from build123d import *

# Parameters (mm, degrees)
F0_W     = 711.2
F0_H     = 254
F1_DEPTH = 457.2
F3_DEPTH = 711.201
F4_R     = 19.05


with BuildPart() as f1:
    # F0 (on Top) → F1 (new body)
    with BuildSketch(Plane.XY):
        Rectangle(F0_W, F0_H)
    extrude(amount=F1_DEPTH)

    # F2 (on face) → F3 (cut, through all)
    with BuildSketch(Plane.YZ.offset(355.6)):
        Polygon((-127, 457.2), (-127, 0), (0, 457.2), align=None)
    extrude(amount=-F3_DEPTH, mode=Mode.SUBTRACT)

    # F4
    f4_edges = [f1.edges().sort_by_distance(p)[0] for p in [
        (0, -127, 0),
        (355.6, 0, 0),
        (355.6, -63.5, 228.6),
        (-355.6, -63.5, 228.6),
        (-355.6, 0, 0),
        (-355.6, 63.5, 457.2),
        (0, 0, 457.2),
        (355.6, 63.5, 457.2),
        (355.6, 127, 228.6),
        (0, 127, 0),
        (-355.6, 127, 228.6),
        (0, 127, 457.2),
    ]]
    fillet(f4_edges, radius=F4_R)


solid = f1.part
The model under review builds one solid part; all positions refer to its coordinate system, in mm. Round coordinates to 2 decimals unless told otherwise and drop trailing zeros. Loops run counter-clockwise (first coordinate to the right, second up) from the corner with the lowest first, then second, coordinate; pieces in that order, holes last. Notation, with made-up numbers: (87.5, 69) -> (107.5, 69) arc R11 ccw to (107.5, 85) -> close; hole circle Ø4 at (63.5, -34.5). An arc over 180 degrees is marked (long way). One line per question, with ' | ' between items. Start each with the question number.
Item 1: Add section A-A, the plane x = -190.5. Write out the cut boundary in (y, z), then the cut area to 3 significant figures.
Item 2: Wall thickness on line 1 along Y through (x, z) = (-286, 288); line 2 along X through (y, z) = (-20.5, 341.5); line 3 along Y through (x, z) = (-143.5, 233): over which ranges is each line inside the solid? List them lowest first. Write a range as [from, to].
Item 3: For pin 1 (6 mm diameter, centred on x = 66, z = 86.5, fed in from -Y); pin 2 (1.5 mm diameter, centred on y = -37.5, z = 309.5, fed in from -X); pin 3 (1.5 mm diameter, centred on x = 122, z = 85.5, fed in from -Y), all flat-tipped, find the tip position at first contact; note any pin that passes through.
Return value:
1) outline: (-120.29, 24.15) arc R19.05 ccw to (-101.94, 0) -> (107.95, 0) arc R19.05 ccw to (127, 19.05) -> (127, 438.15) arc R19.05 ccw to (107.95, 457.2) -> (14.48, 457.2) arc R19.05 ccw to (-3.88, 443.25) -> close | area: 86,800 mm2
2) line 1: y = [-47, 127] | line 2: x = [-353.91, 353.91] | line 3: y = [-62.28, 127]
3) pin 1: stops at y = -103.81 | pin 2: stops at x = -348.42 | pin 3: stops at y = -103.46
